For this review, use the dimensioned drawing (mm, ordinates from the lowest corner) and the shaded views. A direction names the side the tool comes from. Coordinates: 2 decimals unless noted, no trailing zeros. Write each loop counter-clockwise with the first axis right and the second up, starting at its lowest first coordinate (ties: lowest second). Pieces come first, ordered by that corner, then holes. Notation, with made-up numbers: (67, 42.25) - (77, 42.25) arc R14 ccw to (77, 54.25) - close; hole circle Ø4 at (3, 42.25). An arc over 180 degrees is marked (long way). Put each result on its own line as item: value.
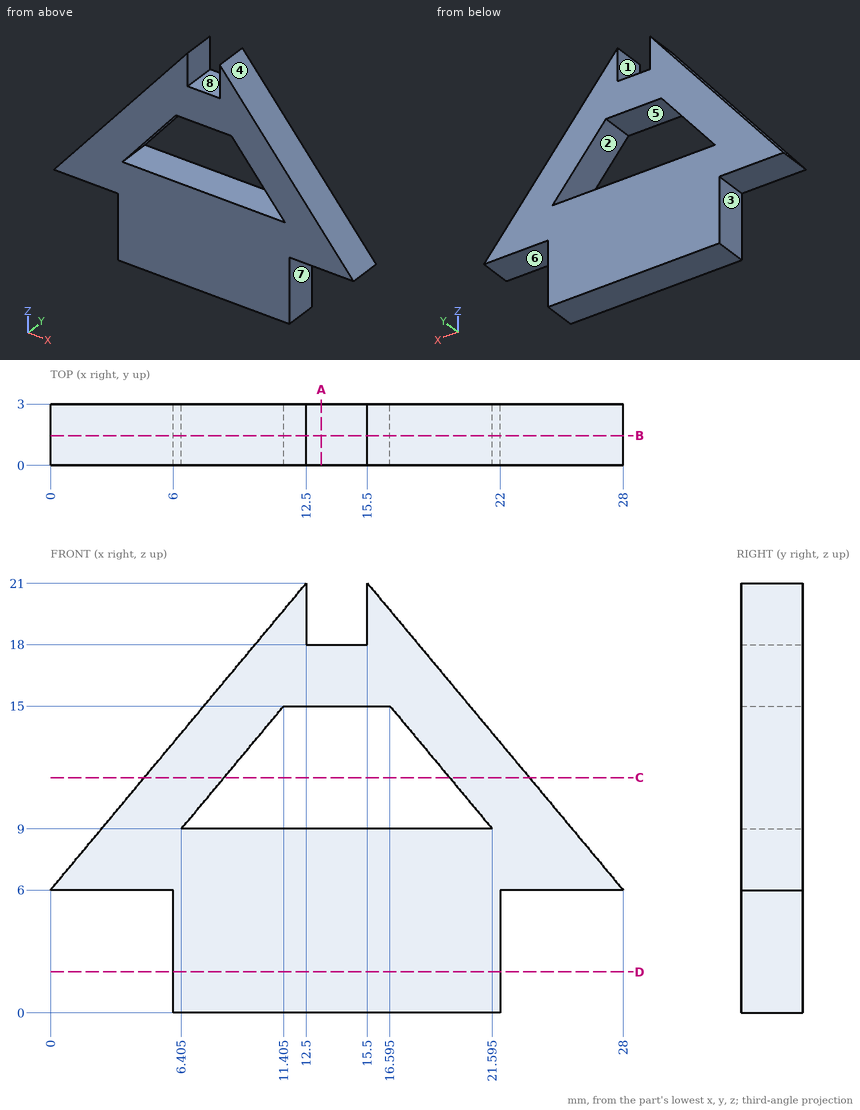
1. Consider section C-C on z = 11.5. State the section outline as (x, y) points, plus the area to 3 significant figures.
Determined:
outline: (4.58, 0) - (8.49, 0) - (8.49, 3) - (4.58, 3) - close; (19.51, 0) - (23.42, 0) - (23.42, 3) - (19.51, 3) - close
area: 23.4 mm^2
2. Consider section A-A on x = 13.25. State the section outline as (y, z) points, plus the area to 3 significant figures.
Determined:
outline: (0, 0) - (3, 0) - (3, 9) - (0, 9) - close; (0, 15) - (3, 15) - (3, 18) - (0, 18) - close
area: 36.0 mm^2
3. Consider section D-D on z = 2. State the section outline as (x, y) points.
Determined:
outline: (6, 0) - (22, 0) - (22, 3) - (6, 3) - close
4. Consider section B-B on y = 1.45. State the section outline as (x, z) points (3 decimals).
Determined:
outline: (0, 6) - (6, 6) - (6, 0) - (22, 0) - (22, 6) - (28, 6) - (15.5, 21) - (15.5, 18) - (12.5, 18) - (12.5, 21) - close; hole (6.405, 9) - (21.595, 9) - (16.595, 15) - (11.405, 15) - close
5. For pin 1 Ø0.9 at (x, y) = (2.5, 2) entering from -Z; pin 2 Ø1.5 at (y, z) = (1, 18) entering from +X (3 decimals); pin 3 Ø1.5 at (x, y) = (12, 2) entering from +Z, all flat-tipped, find the tip position at first contact; note any pin that passes through.
Determined:
pin 1: stops at z = 6
pin 2: stops at x = 18.625
pin 3: stops at z = 21
6. To check wall thickness, follow probe 1 along Z at (x, y) = (15.75, 1.35); probe 2 along X at (y, z) = (2.3, 12) (1 decimal); probe 3 along Z at (x, y) = (19.5, 0.75). State the ranges of each line that lie inside material, in increasing order.
Determined:
probe 1: z = 0 to 9, 15 to 20.7
probe 2: x = 5 to 8.9, 19.1 to 23
probe 3: z = 0 to 9, 11.51 to 16.2
7. The part is to be moulded in two halves that separate along X. For the marked faces 5, 6, 7 and 8, say which applies: +X half, -X half, draft (parallel to the pull), parting line (faces both ways), or undercut.
Determined:
face 5: undercut
face 6: draft
face 7: +X half
face 8: undercut
8. Machinability: for the marked faces 1, 2, 3 and 4, which of the approach directions +Z, -Z, +X, -X, +Y, -Y give a long, thin tool a straight path to every point of the face, cutting with its end or side? Answer none if there is none.
Determined:
face 1: +Z, +Y, -Y
face 2: +Y, -Y
face 3: -Z, -X, +Y, -Y
face 4: +Z, +X, +Y, -Y
